Work out the finished part from the listing and answer in its coordinate system (mm). Round coordinates to 2 decimals unless told otherwise and drop trailing zeros. Use a Markdown table: item, result. Add a question column.
Item 1: For a pull along X with two mould halves and no side action, classify faces 1 (the cylindrical face through (-0.54, 147.9, 2.44)), 2 (the flat face through (2, 300, -2)), 3 (the flat face through (-10, 148, 6)) as +X half, -X half, draft (parallel to the pull), parting line (faces both ways), or undercut.
Item 2: Find the intervals of material crossed by L1, parallel to Z at x = 0, y = 124.5; L2, parallel to X at y = 178, z = 6.5, in increasing order. Write a range as [from, to].
Item 3: Flat-ended cylindrical pins translate along their axes: P1, Ø4, axis at x = -0.5, y = 30, coming from the +Z side; P2, Ø4.5, axis at x = 0, z = 0, coming from the +Y side. Find the tip coordinate at first contact, or state that the pin passes through.
from build123d import *

# Parameters (mm, degrees)
SKETCH1_R           = 2.5
BOSS_EXTRUDE1_DEPTH = 300
FILLET1_R           = 0.5
FILLET2_R           = 1


with BuildPart() as part:
    # Sketch1 → Boss-Extrude1 (new body)
    with BuildSketch(Plane(origin=(0, 0, 0), x_dir=(1, 0, 0), z_dir=(0, 1, 0))):
        with BuildLine():
            Line((3.2, 10), (3.2, 8.6))
            Line((3.2, 8.6), (7.610050506, 8.6))
            Line((7.610050506, 8.6), (2.289805316, 3.27975481))
            ThreePointArc((2.289805316, 3.27975481), (0, 4), (-2.289805316, 3.27975481))
            Line((-2.289805316, 3.27975481), (-7.610050506, 8.6))
            Line((-7.610050506, 8.6), (-3.2, 8.6))
            Line((-3.2, 8.6), (-3.2, 10))
            Line((-3.2, 10), (-10, 10))
            Line((-10, 10), (-10, 3.2))
            Line((-10, 3.2), (-8.6, 3.2))
            Line((-8.6, 3.2), (-8.6, 7.610050506))
            Line((-8.6, 7.610050506), (-3.27975481, 2.289805316))
            ThreePointArc((-3.27975481, 2.289805316), (-4, 0), (-3.27975481, -2.289805316))
            Line((-3.27975481, -2.289805316), (-8.6, -7.610050506))
            Line((-8.6, -7.610050506), (-8.6, -3.2))
            Line((-8.6, -3.2), (-10, -3.2))
            Line((-10, -3.2), (-10, -10))
            Line((-10, -10), (-3.2, -10))
            Line((-3.2, -10), (-3.2, -8.6))
            Line((-3.2, -8.6), (-7.610050506, -8.6))
            Line((-7.610050506, -8.6), (-2.289805316, -3.27975481))
            ThreePointArc((-2.289805316, -3.27975481), (0, -4), (2.289805316, -3.27975481))
            Line((2.289805316, -3.27975481), (7.610050506, -8.6))
            Line((7.610050506, -8.6), (3.2, -8.6))
            Line((3.2, -8.6), (3.2, -10))
            Line((3.2, -10), (10, -10))
            Line((10, -10), (10, -3.2))
            Line((10, -3.2), (8.6, -3.2))
            Line((8.6, -3.2), (8.6, -7.610050506))
            Line((8.6, -7.610050506), (3.27975481, -2.289805316))
            ThreePointArc((3.27975481, -2.289805316), (4, 0), (3.27975481, 2.289805316))
            Line((3.27975481, 2.289805316), (8.6, 7.610050506))
            Line((8.6, 7.610050506), (8.6, 3.2))
            Line((8.6, 3.2), (10, 3.2))
            Line((10, 3.2), (10, 10))
            Line((10, 10), (3.2, 10))
        make_face()
        Circle(SKETCH1_R, mode=Mode.SUBTRACT)
    extrude(amount=BOSS_EXTRUDE1_DEPTH)

    # Fillet1
    fillet1_edges = [part.edges().sort_by_distance(p)[0] for p in [
        (8.6, 150, -7.610050506),
        (8.6, 150, 7.610050506),
        (7.610050506, 150, 8.6),
        (-7.610050506, 150, 8.6),
        (-8.6, 150, 7.610050506),
        (-8.6, 150, -7.610050506),
        (-7.610050506, 150, -8.6),
        (7.610050506, 150, -8.6),
    ]]
    fillet(fillet1_edges, radius=FILLET1_R)

    # Fillet2
    fillet2_edges = [part.edges().sort_by_distance(p)[0] for p in [
        (10, 150, 10),
        (-10, 150, 10),
        (-10, 150, -10),
        (10, 150, -10),
    ]]
    fillet(fillet2_edges, radius=FILLET2_R)


solid = part.part
Reported:
| question | item | result |
|---|---|---|
| 1 | face 1 | undercut |
| 1 | face 2 | draft |
| 1 | face 3 | -X half |
| 2 | L1 | [-4, -2.5], [2.5, 4] |
| 2 | L2 | [-10, -8.59], [-7.49, -5.51], [5.51, 7.49], [8.59, 10] |
| 3 | P1 | z = 4 |
| 3 | P2 | through |
